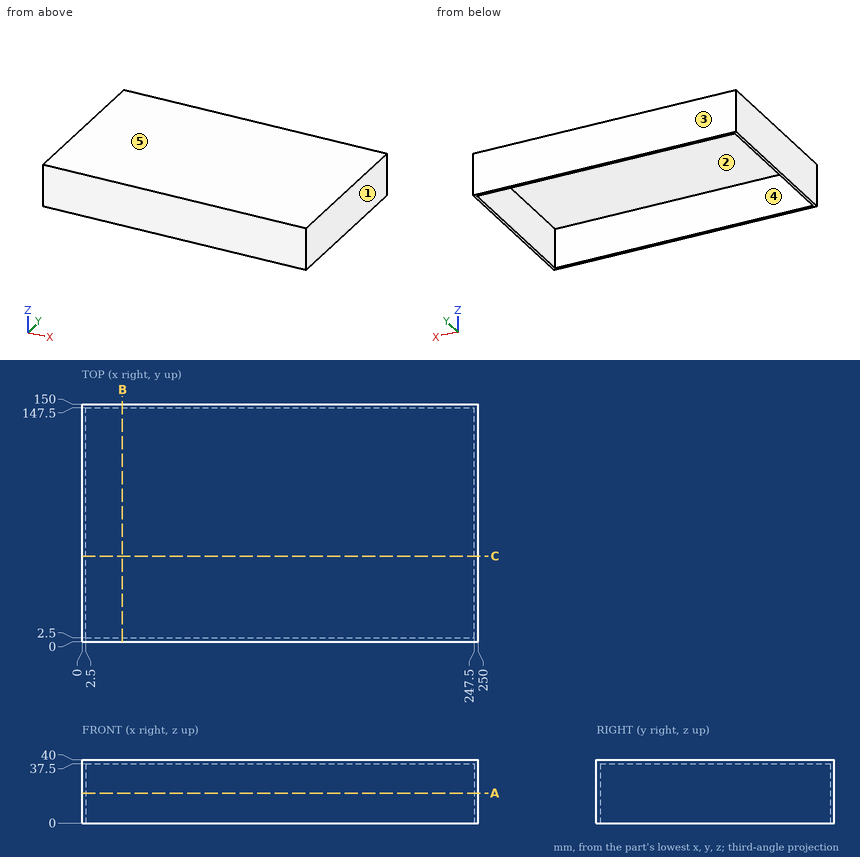
Could you check a few things on this drawing? It's one solid part, dimensions in mm from its lowest x, y, z. A direction names the side the tool comes from. Give positions to 0.01 mm unless a question says otherwise; leave off trailing zeros. Loops run counter-clockwise (first coordinate to the right, second up) from the corner with the lowest first, then second, coordinate; pieces in that order, holes last. Notation, with made-up numbers: (84.25, 13.25) -> (121.25, 13.25) arc R12 ccw to (121.25, 32.25) -> close; hole circle Ø9 at (49, 56). An arc over 180 degrees is marked (long way). Use one line per item in the form item = value. Start each with the question number.
1) For P1, Ø12, axis at x = 25.5, z = 8, coming from the -Y side; P2, Ø3, axis at x = 145, y = 93.5, coming from the -Z side, each with a flat end and sliding along its axis, tell me the tip position at first contact or that it passes through.
2) Imagine slicing it at C-C (y = 54). Please give me the cut outline in (x, z).
3) Imagine slicing it at B-B (x = 25.5). Please give me the cut outline in (y, z).
4) Which directions (+Z, -Z, +X, -X, +Y, -Y) give clear straight access to the entire face, cutting with the end or side of a thin tool? Please do the marked faces 1 and 2.
5) Imagine slicing it at A-A (z = 19). Please give me the cut outline in (x, y).
6) Please list where these lines run through material, in increasing order: line 1 along X through (y, z) = (13, 32); line 2 along Y through (x, z) = (211, 25); line 3 along Z through (x, y) = (21, 112.5).
7) Thinking about a two-plate mould opening in Y: for the marked faces 3, 4 and 5, which applies, +Y half, -Y half, draft (parallel to the pull), parting line (faces both ways), or undercut?
Check values:
q1.P1 = 0
q1.P2 = 37.5
q2.outline = (0, 0) -> (2.5, 0) -> (2.5, 37.5) -> (247.5, 37.5) -> (247.5, 0) -> (250, 0) -> (250, 40) -> (0, 40) -> close
q3.outline = (0, 0) -> (2.5, 0) -> (2.5, 37.5) -> (147.5, 37.5) -> (147.5, 0) -> (150, 0) -> (150, 40) -> (0, 40) -> close
q4.face_1 = +Z, -Z, +X, +Y, -Y
q4.face_2 = -Z
q5.outline = (0, 0) -> (250, 0) -> (250, 150) -> (0, 150) -> close; hole (2.5, 2.5) -> (247.5, 2.5) -> (247.5, 147.5) -> (2.5, 147.5) -> close
q6.line_1 = 0 to 2.5, 247.5 to 250
q6.line_2 = 0 to 2.5, 147.5 to 150
q6.line_3 = 37.5 to 40
q7.face_3 = +Y half
q7.face_4 = undercut
q7.face_5 = draft
